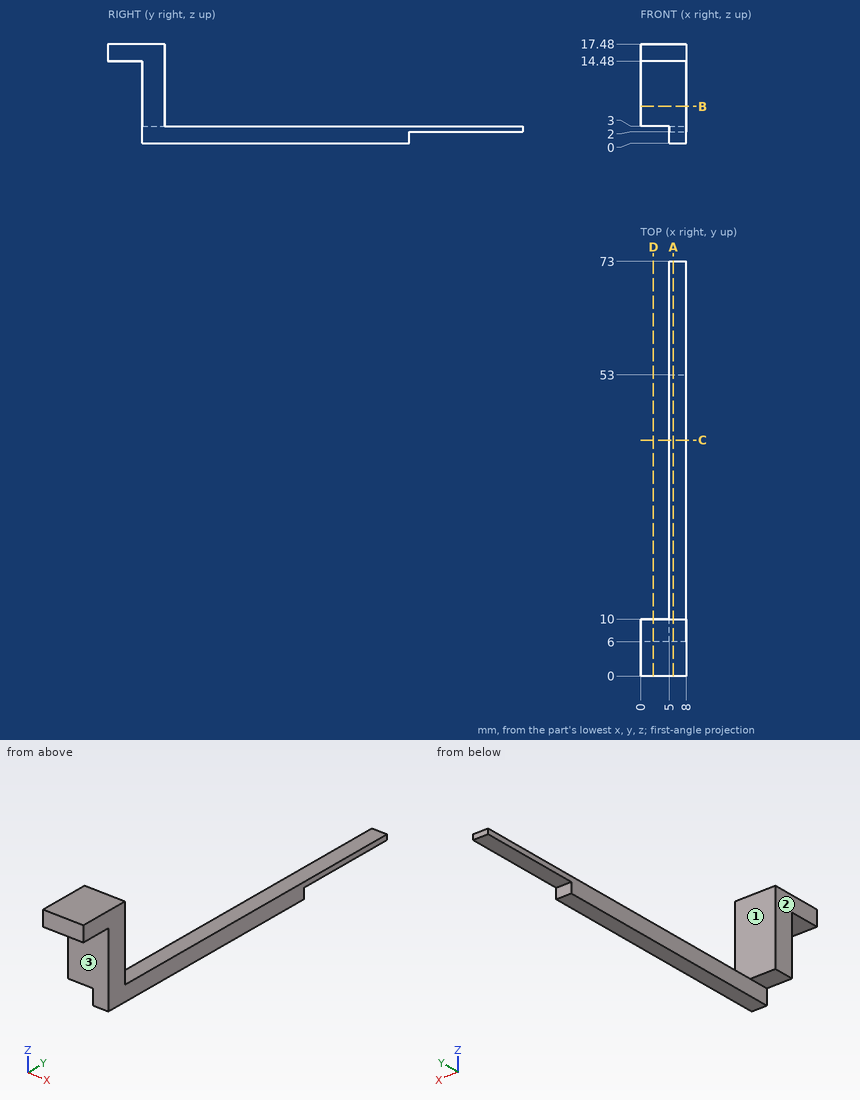
Geometry check sheet. Reference: drawing and pictorial views, mm from the part's lowest x, y, z. A direction names the side the tool comes from. Round coordinates to 2 decimals unless told otherwise and drop trailing zeros. Order: outer loops, then holes, each group sorted by start corner. A loop starts at its lowest first (then second) coordinate and runs counter-clockwise, first axis right, second up. Notation, with made-up numbers: (32.5, 89) - (50.5, 89) arc R20 cw to (50.5, 121) - close; hole circle Ø8 at (48, 50). An arc over 180 degrees is marked (long way). One line per question, with ' | ' between items. Start each with the question number.
(1) Sectioned sample at B-B on z = 6.5. Record the cut outline in (x, y).
(2) Thickness scan on L1, parallel to Y at x = 7.75, z = 2.5; L2, parallel to Z at x = 5.25, y = 38.5; L3, parallel to Y at x = 7.75, z = 4.5. Record the ranges inside material, lowest first. Write a range as [from, to].
(3) Depth check by flat-ended pin: pin 1 Ø4 at (x, y) = (6.5, 53) entering from +Z; pin 2 Ø4 at (x, z) = (2.5, 7.5) entering from -Y; pin 3 Ø5 at (y, z) = (65, 6) entering from +X; pin 4 Ø3 at (x, y) = (1.5, 9) entering from -Z. Enter the tip coordinate at first touch or a pass-through.
(4) Sectioned sample at A-A on x = 5.75. Record the cut outline in (y, z), and give its area (3 significant figures).
(5) Sectioned sample at C-C on y = 41.5. Record the cut outline in (x, z).
(6) Sectioned sample at D-D on x = 2.25. Record the cut outline in (y, z), and give its area (3 significant figures).
(7) Access from +Z, -Z, +X, -X, +Y, -Y to the whole of each face (thin tool, end or side, straight path). Record for the marked faces 1, 2 and 3.
Conclusion:
1) outline: (0, 6) - (8, 6) - (8, 10) - (0, 10) - close
2) L1: y = [6, 73] | L2: z = [0, 3] | L3: y = [6, 10]
3) pin 1: stops at z = 3 | pin 2: stops at y = 6 | pin 3: passes through | pin 4: stops at z = 3
4) outline: (0, 14.48) - (6, 14.48) - (6, 0) - (53, 0) - (53, 2) - (73, 2) - (73, 3) - (10, 3) - (10, 17.48) - (0, 17.48) - close | area: 237 mm2
5) outline: (5, 0) - (8, 0) - (8, 3) - (5, 3) - close
6) outline: (0, 14.48) - (6, 14.48) - (6, 3) - (10, 3) - (10, 17.48) - (0, 17.48) - close | area: 75.9 mm2
7) face 1: +Z, +X, -X, +Y | face 2: +Z, -Z, -X, +Y, -Y | face 3: -Z, +X, -X, -Y
